from build123d import *

# Parameters (mm, degrees)
F0_W     = 57.15
F0_H     = 28.970775
F1_DEPTH = 44.45
F2_R     = 14.717046
F3_R     = 19.003724
F4_DEPTH = 66.548
F5_T     = -2.54
F6_W     = 14.110848
F6_H     = 44.45
F6_R     = 2.9464
F7_DEPTH = 3.81


with BuildPart() as f1:
    # F0 (on Front) → F1 (new body)
    with BuildSketch(Plane.XZ):
        with Locations((-28.575, 14.485387)):
            Rectangle(F0_W, F0_H)
    extrude(amount=F1_DEPTH)

    # F2
    f2_edges = [f1.edges().sort_by_distance(p)[0] for p in [
        (0, -22.225, 28.970775),
    ]]
    fillet(f2_edges, radius=F2_R)

    # F3 (on Front) → F4 (cut)
    with BuildSketch(Plane.XZ):
        Circle(F3_R)
    extrude(amount=F4_DEPTH, mode=Mode.SUBTRACT)

    # F5
    f5_openings = [f1.faces().sort_by_distance(p)[0] for p in [
        (-38.076862, -22.225, 0),
    ]]
    offset(amount=F5_T, openings=f5_openings)

    # F6 (on face) → F7 (join)
    with BuildSketch(Plane(origin=(0, 0, 0), x_dir=(1, 0, 0), z_dir=(0, 0, -1))):
        with Locations((-36.744211, 22.225)):
            Rectangle(F6_W, F6_H)
        with Locations((-36.744211, 22.225)):
            Circle(F6_R, mode=Mode.SUBTRACT)
    extrude(amount=-F7_DEPTH)


solid = f1.part
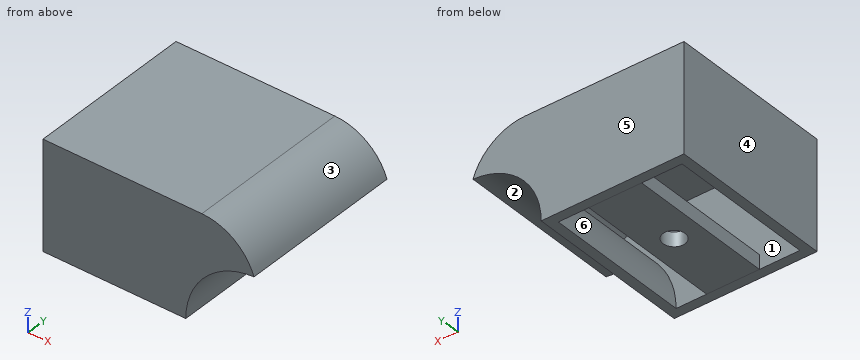
The listing builds one solid part. Answer for the finished solid, in the listing's coordinates (mm). Face numbers are marked on the shaded views. A direction names the side the tool comes from. Round coordinates to 2 decimals unless told otherwise and drop trailing zeros. Order: outer loops, then holes, each group sorted by start corner. A loop starts at its lowest first (then second) coordinate and runs counter-clockwise, first axis right, second up. Notation, with made-up numbers: M 62,25 L 95,25 A25 cw 95,42 Z; hole C 79.5,89 d10. An arc over 180 degrees is marked long. Answer in a Markdown table with one row per item. Add a question column.
1) Consider line 1 along Z through (x, y) = (-39.5, -10.5); line 2 along Y through (x, z) = (-13, 25.5); line 3 along X through (y, z) = (-41, 2.25). Determine where each line is inside the solid, lowest interval first. Write a range as from..to.
2) Which of the six approach directions +Z, -Z, +X, -X, +Y, -Y give full straight-line access (tool end or side, diameter ignored) to the marked faces 5 and 6?
3) The part is cut by section A-A on y = -17. Determine the outline of the cut face in (x, z).
4) The part is cut by section B-B on x = -53. Determine the outline of the cut face in (y, z).
5) The part is cut by section C-C on z = 8.75. Determine the outline of the cut face in (x, y), plus the area to 3 significant figures.
6) Flat-ended cylindrical pins translate along their axes: pin 1 Ø8 at (y, z) = (-24, 10.5) entering from +X; pin 2 Ø3 at (y, z) = (-29, 1) entering from +X. Find the tip coordinate at first contact, or state that the pin passes through.
7) The part is cut by section D-D on x = -9. Determine the outline of the cut face in (y, z).
8) Determine the mould class of the marked faces 1, 2, 3 and 4 for opening direction Z: pulls with the +Z half, pulls with the -Z half, needs draft (parallel to the pull), parting line crosses it, or undercut.
Findings below:
| question | item | result |
|---|---|---|
| 1 | line 1 | z = 0..3.81, 26.43..28.97 |
| 1 | line 2 | y = -44.45..-41.91, -2.54..0 |
| 1 | line 3 | x = -57.15..-54.61, -43.8..-29.69, -21.43..-18.87 |
| 2 | face 5 | +Z, -Z, +X, -X, +Y |
| 2 | face 6 | none |
| 3 | outline | M -57.15,0 L -54.61,0 L -54.61,26.43 L -14.72,26.43 A12.18 cw -4.61,21.04 A21.54 ccw -21.54,0 L -19,0 A19 cw -0.78,18.99 A14.72 ccw -14.72,28.97 L -57.15,28.97 Z; M -43.8,0 L -29.69,0 L -29.69,3.81 L -43.8,3.81 Z |
| 4 | outline | M -44.45,0 L -41.91,0 L -41.91,26.43 L -2.54,26.43 L -2.54,0 L 0,0 L 0,28.97 L -44.45,28.97 Z |
| 5 | outline | M -57.15,-44.45 L -16.87,-44.45 L -16.87,0 L -57.15,0 Z; hole M -54.61,-41.91 L -19.69,-41.91 L -19.69,-2.54 L -54.61,-2.54 Z |
| 5 | area | 416 mm² |
| 6 | pin 1 | stops at x = -12.28 |
| 6 | pin 2 | stops at x = -18.84 |
| 7 | outline | M -44.45,16.74 L 0,16.74 L 0,27.81 L -44.45,27.81 Z; hole M -41.91,19.57 L -2.54,19.57 L -2.54,25.01 L -41.91,25.01 Z |
| 8 | face 1 | undercut |
| 8 | face 2 | pulls with the -Z half |
| 8 | face 3 | pulls with the +Z half |
| 8 | face 4 | needs draft |
